```python
from build123d import *

# Parameters (mm, degrees)
ESQUISSE1_W                                   = 60
ESQUISSE1_H                                   = 190
BOSS_EXTRU_1_DEPTH                            = 20
TROU_POUR_TARAUDAGE_POUR_TROU_TARAUD_M6_D     = 5
TROU_POUR_TARAUDAGE_POUR_TROU_TARAUD_M6_DEPTH = 15
TROU_POUR_TARAUDAGE_POUR_TROU_TARAUD_M6_TIP   = 1.502151548
D_GAGEMENT_M61_D                              = 6.2
R_P_TITION_LIN_AIRE1_COUNT                    = 13
R_P_TITION_LIN_AIRE1_PITCH                    = 12.5


with BuildPart() as part:
    # Esquisse1 → Boss.-Extru.1 (new body)
    with BuildSketch(Plane.XY):
        Rectangle(ESQUISSE1_W, ESQUISSE1_H)
    extrude(amount=BOSS_EXTRU_1_DEPTH)

    # Trou pour taraudage pour trou taraudé M61
    with Locations(Plane(origin=(0, -95, 0), x_dir=(-1, 0, 0), z_dir=(0, -1, 0))):
        with Locations((-20, -10), (20, -10)):
            Hole(TROU_POUR_TARAUDAGE_POUR_TROU_TARAUD_M6_D / 2, depth=TROU_POUR_TARAUDAGE_POUR_TROU_TARAUD_M6_DEPTH)
            with Locations((0, 0, -(TROU_POUR_TARAUDAGE_POUR_TROU_TARAUD_M6_DEPTH + TROU_POUR_TARAUDAGE_POUR_TROU_TARAUD_M6_TIP / 2))):  # 118° drill point
                Cone(0, TROU_POUR_TARAUDAGE_POUR_TROU_TARAUD_M6_D / 2, TROU_POUR_TARAUDAGE_POUR_TROU_TARAUD_M6_TIP, mode=Mode.SUBTRACT)

    # Dégagement M61 (through all)
    with Locations(Plane.XY.offset(20)):
        with Locations((-16, -65), (16, -65)):
            d_gagement_m61 = Hole(D_GAGEMENT_M61_D / 2)

    # Répétition linéaire1: Dégagement M61 ×13
    with Locations(*[(0, i * R_P_TITION_LIN_AIRE1_PITCH, 0) for i in range(1, R_P_TITION_LIN_AIRE1_COUNT)]):
        add(d_gagement_m61, mode=Mode.SUBTRACT)


solid = part.part
```
Geometry check sheet. Reference: the model listing, model coordinates, mm. A direction names the side the tool comes from. Give positions to 0.01 mm unless a question says otherwise; leave off trailing zeros. Order: outer loops, then holes, each group sorted by start corner. A loop starts at its lowest first (then second) coordinate and runs counter-clockwise, first axis right, second up. Notation, with made-up numbers: (-36, 16) - (-22, 16) arc R25 ccw to (-22, 51) - close; hole circle Ø11 at (3.25, 29). An arc over 180 degrees is marked (long way). Write item = value, one per line. Start each with the question number.
1) Access from +Z, -Z, +X, -X, +Y, -Y to the whole of each face (thin tool, end or side, straight path). Record for faces 1 (the cylindrical face through (18, -87.4, 11.5)), 2 (the cylindrical face through (14.57, 19.75, 9.86)).
2) Section check A-A (y = 60). Enter the section's corners in (x, z), then the cut area to 3 significant figures.
3) Gauge pin test, flat end, axial feed: pin 1 Ø4.5 at (x, z) = (-20, 10) entering from -Y. Record the tip position at first contact, or that the pin passes through.
4) Draft check along X on faces 3 (the cylindrical face through (-22, -87.4, 11.5)), 4 (the flat face through (30, -1, 10)), 5 (the flat face through (0, 95, 10)). Enter one of: released by +X, released by -X, zero draft, split by the parting line, or undercut.
5) Section check B-B (z = 15.5). Count the separate pieces of the cut face and the enclosed holes in it, then the cut area to 3 significant figures.
6) Scan line: L1, parallel to X at y = 11, z = 11. Record every from-to range of solid material in increasing order.
Geometry check:
q1.face_1 = -Y
q1.face_2 = +Z, -Z
q2.outline = (-30, 0) - (-19.1, 0) - (-19.1, 20) - (-30, 20) - close; (-12.9, 0) - (12.9, 0) - (12.9, 20) - (-12.9, 20) - close; (19.1, 0) - (30, 0) - (30, 20) - (19.1, 20) - close
q2.area = 952 mm2
q3.pin_1 = -79.85
q4.face_3 = undercut
q4.face_4 = released by +X
q4.face_5 = zero draft
q5.separate_pieces = 1
q5.enclosed_holes = 26
q5.area = 10,600 mm2
q6.L1 = -30 to -18.93, -13.07 to 13.07, 18.93 to 30
